from build123d import *

# Parameters (mm, degrees)
BOSS_EXTRUDE1_DEPTH = 16
FILLET1_R           = 16
SKETCH6_R           = 7
CUT_EXTRUDE3_DEPTH  = 14
SKETCH3_R           = 8
CUT_EXTRUDE2_DEPTH  = 18


with BuildPart() as part:
    # Sketch1 → Boss-Extrude1 (new, symmetric)
    with BuildSketch(Plane.XY):
        Polygon((36, 0), (-36, 0), (-36, 14), (-9, 14), (-9, 46), (9, 46), (9, 14), (36, 14), align=None)
    extrude(amount=BOSS_EXTRUDE1_DEPTH, both=True)

    # Fillet1
    fillet1_edges = [part.edges().sort_by_distance(p)[0] for p in [
        (0, 46, -16),
        (0, 46, 16),
    ]]
    fillet(fillet1_edges, radius=FILLET1_R - 0.0001)  # a hair under: the kernel refuses the full size

    # Sketch6 → Cut-Extrude3 (cut)
    with BuildSketch(Plane(origin=(0, 14, 0), x_dir=(1, 0, 0), z_dir=(0, 1, 0))):
        with Locations(Location((-24, 0, 0), (0, 0, 180))):
            Circle(SKETCH6_R)
        with Locations((24, 0)):
            Circle(SKETCH6_R)
    extrude(amount=-CUT_EXTRUDE3_DEPTH, mode=Mode.SUBTRACT)

    # Sketch3 → Cut-Extrude2 (cut)
    with BuildSketch(Plane(origin=(9, 0, 0), x_dir=(0, 0, -1), z_dir=(1, 0, 0))):
        with Locations((0, 29)):
            Circle(SKETCH3_R)
    extrude(amount=-CUT_EXTRUDE2_DEPTH, mode=Mode.SUBTRACT)


solid = part.part
Design review of the part built by this model. Coordinates are the model's own, in mm. A direction names the side the tool comes from. Give positions to 0.01 mm unless a question says otherwise; leave off trailing zeros. Write each loop counter-clockwise with the first axis right and the second up, starting at its lowest first coordinate (ties: lowest second). Pieces come first, ordered by that corner, then holes. Notation, with made-up numbers: M 68.5,14 L 90.5,14 A36 cw 90.5,50 Z; hole C 17.5,87 d10. An arc over 180 degrees is marked long. Return JSON: item names as keys, results as strings. Group by question number.
Item 1: Tool access review of faces 5 (the flat face through (-16.7, 14, 0.2)), 6 (the flat face through (-36, 7, 0)), 7 (the flat face through (9, 34, -7)): name each direction out of +Z, -Z, +X, -X, +Y, -Y from which nothing blocks a thin tool from reaching the whole face with its end or side.
Item 2: Wall thickness on line 1 along X through (y, z) = (8, 0.5); line 2 along Y through (x, z) = (-2, 0); line 3 along Z through (x, y) = (-24, 8): over which ranges is each line inside the solid? List them lowest first.
Item 3: Take a section at C-C (z = -3). Give the boundary of the cut face in (x, y), plus the area to 3 significant figures.
Item 4: Take a section at A-A (x = 24). Give the boundary of the cut face in (y, z).
Item 5: The part is to be moulded in two halves that separate along Z. For faces 1 (the cylindrical face through (0.126, 41.437, -11.189)), 2 (the cylindrical face through (0.126, 36.932, 1.041)), 3 (the flat face through (-9, 33.3, 7.3)), 4 (the flat face through (1, 12, 16)), say which applies: pulls with the +Z half, pulls with the -Z half, needs draft (parallel to the pull), parting line crosses it, or undercut.
Item 6: Clearance check with flat-ended pins moving along their axes: pin 1 Ø1 at (x, z) = (-8.5, 8.5) entering from +Y; pin 2 Ø11 at (x, z) = (24, 0) entering from -Y; pin 3 Ø9.5 at (y, z) = (29.5, -3.5) entering from -X; pin 4 Ø10 at (y, z) = (35, -2) entering from +X. State where each tip first meets the part, or that it passes through.
Item 7: Take a section at B-B (y = 29). Give the boundary of the cut face in (x, z).
Return value:
{
 "1": {"face 5": "+Z, -Z, -X, +Y", "face 6": "+Z, -Z, -X, +Y, -Y", "face 7": "+Z, -Z, +X, +Y"},
 "2": {"line 1": "x = -36 to -30.98, -17.02 to 17.02, 30.98 to 36", "line 2": "y = 0 to 21, 37 to 46", "line 3": "z = -16 to -7, 7 to 16"},
 "3": {"outline": "M -36,0 L -30.32,0 L -30.32,14 L -36,14 Z; M -17.68,0 L 17.68,0 L 17.68,14 L 9,14 L 9,21.58 L -9,21.58 L -9,14 L -17.68,14 Z; M -9,36.42 L 9,36.42 L 9,45.72 L -9,45.72 Z; M 30.32,0 L 36,0 L 36,14 L 30.32,14 Z", "area": "958 mm2"},
 "4": {"outline": "M 0,-16 L 14,-16 L 14,-7 L 0,-7 Z; M 0,7 L 14,7 L 14,16 L 0,16 Z"},
 "5": {"face 1": "pulls with the -Z half", "face 2": "undercut", "face 3": "needs draft", "face 4": "pulls with the +Z half"},
 "6": {"pin 1": "stops at y = 43.86", "pin 2": "passes through", "pin 3": "stops at x = -9", "pin 4": "stops at x = 9"},
 "7": {"outline": "M -9,-16 L 9,-16 L 9,-8 L -9,-8 Z; M -9,8 L 9,8 L 9,16 L -9,16 Z"}
}
